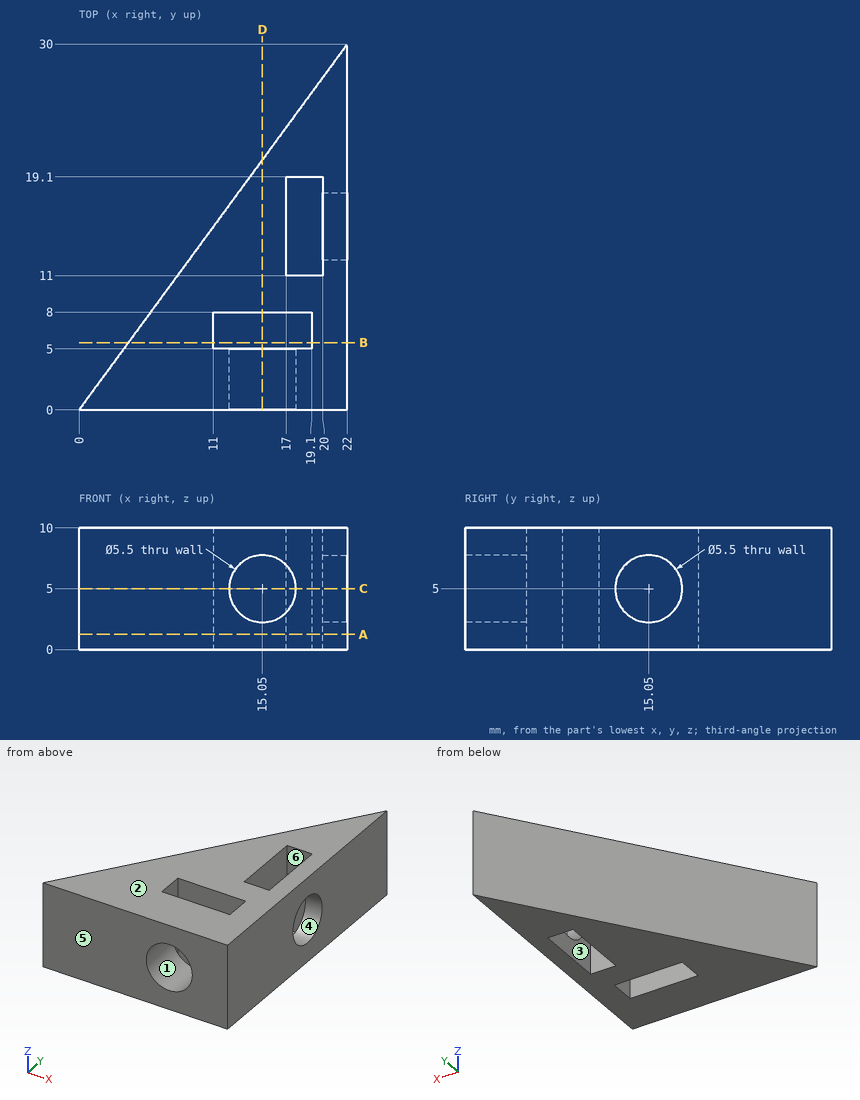
Geometry check sheet. Reference: drawing and pictorial views, mm from the part's lowest x, y, z. A direction names the side the tool comes from. Give positions to 0.01 mm unless a question says otherwise; leave off trailing zeros. Order: outer loops, then holes, each group sorted by start corner. A loop starts at its lowest first (then second) coordinate and runs counter-clockwise, first axis right, second up. Notation, with made-up numbers: M 42,89.25 L 53,89.25 A19 cw 53,95.25 Z; hole C -15,87 d9. An arc over 180 degrees is marked long. Answer in a Markdown table with one row per item. Add a question column.
Q1. Release check for a two-part mould opening along Z. For the marked faces 1, 2 and 3 record: released by +Z, released by -Z, zero draft, split by the parting line, or undercut.
Q2. Gauge pin test, flat ends, axial feed: pin 1 Ø3 at (x, z) = (11, 4.5) entering from +Y; pin 2 Ø3.5 at (y, z) = (15.05, 5) entering from +X; pin 3 Ø5 at (x, y) = (8.5, 11.5) entering from -Z; pin 4 Ø4 at (x, z) = (14, 5.5) entering from +Y. Record the tip position at first contact, or that the pin passes through.
Q3. Sectioned sample at D-D, the plane x = 15.05. Record the boundary of the cut face in (y, z), and give its area (3 significant figures).
Q4. Sectioned sample at A-A, the plane z = 1.25. Record the boundary of the cut face in (x, y), and give its area (3 significant figures).
Q5. Access from +Z, -Z, +X, -X, +Y, -Y to the whole of each face (thin tool, end or side, straight path). Record for the marked faces 4, 5 and 6.
Q6. Sectioned sample at C-C, the plane z = 5. Record the boundary of the cut face in (x, y).
Q7. Sectioned sample at B-B, the plane y = 5.5. Record the boundary of the cut face in (x, z).
Q8. Thickness scan on L1, parallel to Z at x = 15.05, y = 3.65; L2, parallel to X at y = 18.5, z = 4.5; L3, parallel to Y at x = 11.5, z = 6. Record the ranges inside material, lowest first.
Verdict:
| question | item | result |
|---|---|---|
| 1 | face 1 | undercut |
| 1 | face 2 | released by +Z |
| 1 | face 3 | zero draft |
| 2 | pin 1 | y = 17.05 |
| 2 | pin 2 | x = 17 |
| 2 | pin 3 | z = 0 |
| 2 | pin 4 | y = 21.82 |
| 3 | outline | M 0,0 L 5,0 L 5,2.25 L 0,2.25 Z; M 0,7.75 L 5,7.75 L 5,10 L 0,10 Z; M 8,0 L 20.52,0 L 20.52,10 L 8,10 Z |
| 3 | area | 148 mm² |
| 4 | outline | M 0,0 L 22,0 L 22,30 Z; hole M 11,5 L 19.1,5 L 19.1,8 L 11,8 Z; hole M 17,11 L 20,11 L 20,19.1 L 17,19.1 Z |
| 4 | area | 281 mm² |
| 5 | face 4 | +X |
| 5 | face 5 | +Z, -Z, +X, -X, -Y |
| 5 | face 6 | +Z, -Z |
| 6 | outline | M 0,0 L 12.3,0 L 12.3,5 L 11,5 L 11,8 L 19.1,8 L 19.1,5 L 17.8,5 L 17.8,0 L 22,0 L 22,12.3 L 20,12.3 L 20,11 L 17,11 L 17,19.1 L 20,19.1 L 20,17.8 L 22,17.8 L 22,30 Z |
| 7 | outline | M 4.03,0 L 11,0 L 11,10 L 4.03,10 Z; M 19.1,0 L 22,0 L 22,10 L 19.1,10 Z |
| 8 | L1 | 0 to 2.25, 7.75 to 10 |
| 8 | L2 | 13.57 to 17, 20 to 22 |
| 8 | L3 | 0 to 5, 8 to 15.68 |
